from build123d import *

# Parameters (mm, degrees)
F0_W         = 150
F0_H         = 80
F1_DEPTH     = 1.5
F2_R         = 2.5
F3_DEPTH     = 30
F4_R         = 1.5
F5_R         = 1.5
F6_R         = 1.5
F7_R         = 1.5
F8_DEPTH     = 25
F9_R         = 1.5
F9_W         = 21
F9_H         = 31
F10_DEPTH    = 3
F12_T1_DEPTH = 1.5


# Not quite as in the source:
# - a fillet or chamfer that OpenCascade refuses, or shapes differently, is made with other operations: its cross-section is extruded or revolved along the edge and cut away or added


with BuildPart() as f1:
    # F0 (on Front) → F1 (new body)
    with BuildSketch(Plane.XZ):
        Rectangle(F0_W, F0_H)
    extrude(amount=F1_DEPTH)

    # F2 (on face) → F3 (join)
    with BuildSketch(Plane(origin=(0, 0, 0), x_dir=(-1, 0, 0), z_dir=(0, 1, 0))):
        with Locations((-25.5, 31)):
            Circle(F2_R)
        with Locations((-25.5, -31)):
            Circle(F2_R)
        with Locations((25.5, -31)):
            Circle(F2_R)
        with Locations((25.5, 31)):
            Circle(F2_R)
    extrude(amount=F3_DEPTH)

    # F4 (on face) + F5 (on face) + F6 (on face) + F7 (on face) → F8 (cut)
    with BuildSketch(Plane(origin=(0, 30, 0), x_dir=(-1, 0, 0), z_dir=(0, 1, 0))):
        with Locations((-25.5, 31)):
            Circle(F4_R)
    with BuildSketch(Plane(origin=(0, 30, 0), x_dir=(-1, 0, 0), z_dir=(0, 1, 0))):
        with Locations((25.5, 31)):
            Circle(F5_R)
    with BuildSketch(Plane(origin=(0, 30, 0), x_dir=(-1, 0, 0), z_dir=(0, 1, 0))):
        with Locations((-25.5, -31)):
            Circle(F6_R)
    with BuildSketch(Plane(origin=(0, 30, 0), x_dir=(-1, 0, 0), z_dir=(0, 1, 0))):
        with Locations((25.5, -31)):
            Circle(F7_R)
    extrude(amount=-F8_DEPTH, mode=Mode.SUBTRACT)

    # F9 (on face) → F10 (cut)
    with BuildSketch(Plane.XZ.offset(1.5)):
        with Locations((-70.5, 0)):
            Circle(F9_R)
        with Locations((-38, 0)):
            Rectangle(F9_W, F9_H)
        with Locations((-13, 0)):
            Rectangle(F9_W, F9_H)
    f10 = extrude(amount=-F10_DEPTH, mode=Mode.SUBTRACT)

    # F11: F10 across plane
    add(f10.mirror(Plane.YZ), mode=Mode.SUBTRACT)

    # F12: fillet of radius 10 on 16 edges, made by hand

    # F12_s2 → F12_t1 (join)
    with BuildSketch(Plane.XZ):
        with BuildLine():
            add(Edge.make_bspline(
                [(-38.5, 15.5), (-48.5, 15.5), (-48.5, 5.5)],
                knots=[0, 0, 0, 1, 1, 1], degree=2, weights=[1, 1.2222222222, 1]))
            Line((-48.5, 5.5), (-48.5, 15.5))
            Line((-48.5, 15.5), (-38.5, 15.5))
        make_face()
        with BuildLine():
            add(Edge.make_bspline(
                [(-37.5, 15.5), (-27.5, 15.5), (-27.5, 5.5)],
                knots=[0, 0, 0, 1, 1, 1], degree=2, weights=[1, 1.2222222222, 1]))
            Line((-27.5, 5.5), (-27.5, 15.5))
            Line((-27.5, 15.5), (-37.5, 15.5))
        make_face()
        with BuildLine():
            add(Edge.make_bspline(
                [(-48.5, -5.5), (-48.5, -15.5), (-38.5, -15.5)],
                knots=[0, 0, 0, 1, 1, 1], degree=2, weights=[1, 1.2222222222, 1]))
            Line((-38.5, -15.5), (-48.5, -15.5))
            Line((-48.5, -15.5), (-48.5, -5.5))
        make_face()
        with BuildLine():
            add(Edge.make_bspline(
                [(-27.5, -5.5), (-27.5, -15.5), (-37.5, -15.5)],
                knots=[0, 0, 0, 1, 1, 1], degree=2, weights=[1, 1.2222222222, 1]))
            Line((-37.5, -15.5), (-27.5, -15.5))
            Line((-27.5, -15.5), (-27.5, -5.5))
        make_face()
        with BuildLine():
            add(Edge.make_bspline(
                [(-2.5, -5.5), (-2.5, -15.5), (-12.5, -15.5)],
                knots=[0, 0, 0, 1, 1, 1], degree=2, weights=[1, 1.2222222222, 1]))
            Line((-12.5, -15.5), (-2.5, -15.5))
            Line((-2.5, -15.5), (-2.5, -5.5))
        make_face()
        with BuildLine():
            add(Edge.make_bspline(
                [(-13.5, 15.5), (-23.5, 15.5), (-23.5, 5.5)],
                knots=[0, 0, 0, 1, 1, 1], degree=2, weights=[1, 1.2222222222, 1]))
            Line((-23.5, 5.5), (-23.5, 15.5))
            Line((-23.5, 15.5), (-13.5, 15.5))
        make_face()
        with BuildLine():
            add(Edge.make_bspline(
                [(-23.5, -5.5), (-23.5, -15.5), (-13.5, -15.5)],
                knots=[0, 0, 0, 1, 1, 1], degree=2, weights=[1, 1.2222222222, 1]))
            Line((-13.5, -15.5), (-23.5, -15.5))
            Line((-23.5, -15.5), (-23.5, -5.5))
        make_face()
        with BuildLine():
            add(Edge.make_bspline(
                [(-12.5, 15.5), (-2.5, 15.5), (-2.5, 5.5)],
                knots=[0, 0, 0, 1, 1, 1], degree=2, weights=[1, 1.2222222222, 1]))
            Line((-2.5, 5.5), (-2.5, 15.5))
            Line((-2.5, 15.5), (-12.5, 15.5))
        make_face()
        with BuildLine():
            add(Edge.make_bspline(
                [(23.5, 5.5), (23.5, 15.5), (13.5, 15.5)],
                knots=[0, 0, 0, 1, 1, 1], degree=2, weights=[1, 1.2222222222, 1]))
            Line((13.5, 15.5), (23.5, 15.5))
            Line((23.5, 15.5), (23.5, 5.5))
        make_face()
        with BuildLine():
            add(Edge.make_bspline(
                [(48.5, 5.5), (48.5, 15.5), (38.5, 15.5)],
                knots=[0, 0, 0, 1, 1, 1], degree=2, weights=[1, 1.2222222222, 1]))
            Line((38.5, 15.5), (48.5, 15.5))
            Line((48.5, 15.5), (48.5, 5.5))
        make_face()
        with BuildLine():
            add(Edge.make_bspline(
                [(2.5, -5.5), (2.5, -15.5), (12.5, -15.5)],
                knots=[0, 0, 0, 1, 1, 1], degree=2, weights=[1, 1.2222222222, 1]))
            Line((12.5, -15.5), (2.5, -15.5))
            Line((2.5, -15.5), (2.5, -5.5))
        make_face()
        with BuildLine():
            add(Edge.make_bspline(
                [(27.5, -5.5), (27.5, -15.5), (37.5, -15.5)],
                knots=[0, 0, 0, 1, 1, 1], degree=2, weights=[1, 1.2222222222, 1]))
            Line((37.5, -15.5), (27.5, -15.5))
            Line((27.5, -15.5), (27.5, -5.5))
        make_face()
        with BuildLine():
            add(Edge.make_bspline(
                [(27.5, 5.5), (27.5, 15.5), (37.5, 15.5)],
                knots=[0, 0, 0, 1, 1, 1], degree=2, weights=[1, 1.2222222222, 1]))
            Line((37.5, 15.5), (27.5, 15.5))
            Line((27.5, 15.5), (27.5, 5.5))
        make_face()
        with BuildLine():
            add(Edge.make_bspline(
                [(2.5, 5.5), (2.5, 15.5), (12.5, 15.5)],
                knots=[0, 0, 0, 1, 1, 1], degree=2, weights=[1, 1.2222222222, 1]))
            Line((12.5, 15.5), (2.5, 15.5))
            Line((2.5, 15.5), (2.5, 5.5))
        make_face()
        with BuildLine():
            add(Edge.make_bspline(
                [(38.5, -15.5), (48.5, -15.5), (48.5, -5.5)],
                knots=[0, 0, 0, 1, 1, 1], degree=2, weights=[1, 1.2222222222, 1]))
            Line((48.5, -5.5), (48.5, -15.5))
            Line((48.5, -15.5), (38.5, -15.5))
        make_face()
        with BuildLine():
            add(Edge.make_bspline(
                [(13.5, -15.5), (23.5, -15.5), (23.5, -5.5)],
                knots=[0, 0, 0, 1, 1, 1], degree=2, weights=[1, 1.2222222222, 1]))
            Line((23.5, -5.5), (23.5, -15.5))
            Line((23.5, -15.5), (13.5, -15.5))
        make_face()
    extrude(amount=F12_T1_DEPTH)


solid = f1.part
Could you check a few things on this model? Use its own coordinates, in mm. A direction names the side the tool comes from. Round coordinates to 2 decimals unless told otherwise and drop trailing zeros. Order: outer loops, then holes, each group sorted by start corner. A loop starts at its lowest first (then second) coordinate and runs counter-clockwise, first axis right, second up.
(1) Imagine slicing it at A-A (y = 21.5). Write out the boundary of the cut face in (x, z), plus the area to 3 significant figures.
Response values:
outline: circle Ø5 at (-25.5, -31); circle Ø5 at (-25.5, 31); circle Ø5 at (25.5, -31); circle Ø5 at (25.5, 31); hole circle Ø3 at (-25.5, -31); hole circle Ø3 at (-25.5, 31); hole circle Ø3 at (25.5, -31); hole circle Ø3 at (25.5, 31)
area: 50.3 mm2
(2) Please list where these lines run through material, in increasing order: line 1 along Z through (x, y) = (25.5, 11.75); line 2 along Z through (x, y) = (-70.5, -0.35); line 3 along X through (y, z) = (11, 33).
Response values:
line 1: z = -33.5 to -32.5, -29.5 to -28.5, 28.5 to 29.5, 32.5 to 33.5
line 2: z = -40 to -1.5, 1.5 to 40
line 3: x = -27 to -24, 24 to 27
(3) If we mould it in two halves opening along Z, with no side actions, what happens to faces 3 (the flat face through (24, 30, 30)), 4 (the cylindrical face through (27, 15, 33)), 5 (the cylindrical face through (69, -1, 0))? For each: released by +Z, released by -Z, zero draft, split by the parting line, or undercut.
Response values:
face 3: zero draft
face 4: undercut
face 5: undercut
(4) Imagine slicing it at D-D (z = -31). Write out the boundary of the cut face in (x, y), plus the area to 3 significant figures.
Response values:
outline: (-75, -1.5) - (75, -1.5) - (75, 0) - (28, 0) - (28, 30) - (27, 30) - (27, 5) - (24, 5) - (24, 30) - (23, 30) - (23, 0) - (-23, 0) - (-23, 30) - (-24, 30) - (-24, 5) - (-27, 5) - (-27, 30) - (-28, 30) - (-28, 0) - (-75, 0) - close
area: 375 mm2
(5) I'm going to push flat-ended pins straight in: pin 1 (0.9 mm diameter, centred on x = -25, z = -31, fed in from +Y); pin 2 (2.5 mm diameter, centred on x = -70.5, z = 0, fed in from -Y); pin 3 (6 mm diameter, centred on x = 12.5, z = 31.5, fed in from +Y). Where does each tip first touch, or does it pass through?
Response values:
pin 1: stops at y = 5
pin 2: passes through
pin 3: stops at y = 0
(6) Which directions (+Z, -Z, +X, -X, +Y, -Y) give clear straight access to the entire face, cutting with the end or side of a thin tool? Please do faces 1 (the flat face through (26, 5, 31)), 2 (the flat face through (24, 30, -32)).
Response values:
face 1: +Y
face 2: +Z, -Z, +X, -X, +Y
(7) Imagine slicing it at B-B (x = 70.5). Write out the boundary of the cut face in (y, z).
Response values:
outline: (-1.5, -40) - (0, -40) - (0, -1.5) - (-1.5, -1.5) - close; (-1.5, 1.5) - (0, 1.5) - (0, 40) - (-1.5, 40) - close
(8) Imagine slicing it at C-C (z = 0). Write out the boundary of the cut face in (x, y).
Response values:
outline: (-75, -1.5) - (-72, -1.5) - (-72, 0) - (-75, 0) - close; (-69, -1.5) - (-48.5, -1.5) - (-48.5, 0) - (-69, 0) - close; (-27.5, -1.5) - (-23.5, -1.5) - (-23.5, 0) - (-27.5, 0) - close; (-2.5, -1.5) - (2.5, -1.5) - (2.5, 0) - (-2.5, 0) - close; (23.5, -1.5) - (27.5, -1.5) - (27.5, 0) - (23.5, 0) - close; (48.5, -1.5) - (69, -1.5) - (69, 0) - (48.5, 0) - close; (72, -1.5) - (75, -1.5) - (75, 0) - (72, 0) - close
